```python
from build123d import *

# Parameters (mm, degrees)
ESBO_O1_W                = 50
ESBO_O1_H                = 62
RESSALTO_EXTRUS_O2_DEPTH = 6
ESBO_O3_W                = 10
ESBO_O3_H                = 6
CORTE_EXTRUS_O1_DEPTH    = 6
ESBO_O4_W                = 10
ESBO_O4_H                = 6
CORTE_EXTRUS_O2_DEPTH    = 6
ESBO_O5_W                = 6
ESBO_O5_H                = 10
CORTE_EXTRUS_O3_DEPTH    = 6


with BuildPart() as part:
    # Esboço1 → Ressalto-extrusão2 (new body)
    with BuildSketch(Plane(origin=(0, 0, 0), x_dir=(1, 0, 0), z_dir=(0, 1, 0))):
        Rectangle(ESBO_O1_W, ESBO_O1_H)
    extrude(amount=RESSALTO_EXTRUS_O2_DEPTH)

    # Esboço3 → Corte-extrusão1 (cut)
    with BuildSketch(Plane.XY.offset(31)):
        with Locations((0, 3)):
            Rectangle(ESBO_O3_W, ESBO_O3_H)
    extrude(amount=-CORTE_EXTRUS_O1_DEPTH, mode=Mode.SUBTRACT)

    # Esboço4 → Corte-extrusão2 (cut)
    with BuildSketch(Plane(origin=(0, 0, -31), x_dir=(-1, 0, 0), z_dir=(0, 0, -1))):
        with Locations((0, 3)):
            Rectangle(ESBO_O4_W, ESBO_O4_H)
    extrude(amount=-CORTE_EXTRUS_O2_DEPTH, mode=Mode.SUBTRACT)

    # Esboço5 → Corte-extrusão3 (cut)
    with BuildSketch(Plane(origin=(0, 6, 0), x_dir=(1, 0, 0), z_dir=(0, 1, 0))):
        Rectangle(ESBO_O5_W, ESBO_O5_H)
    extrude(amount=-CORTE_EXTRUS_O3_DEPTH, mode=Mode.SUBTRACT)


solid = part.part
```
Model file for the job. Use its own axes, mm. A direction names the side the tool comes from. Give positions to 0.01 mm unless a question says otherwise; leave off trailing zeros. Write each loop counter-clockwise with the first axis right and the second up, starting at its lowest first coordinate (ties: lowest second). Pieces come first, ordered by that corner, then holes. Notation, with made-up numbers: (56.25, 7.5) -> (96.25, 7.5) arc R8 ccw to (96.25, 15.5) -> close; hole circle Ø5 at (-19.75, -13.75). An arc over 180 degrees is marked (long way). Use CSV: the item, a comma, the result in double quotes. Start each with the question number.
1) Pin check, flat tips, straight feed: P1, Ø3, axis at x = -2.5, y = 4.5, coming from the -Z side; P2, Ø1.8, axis at x = 0.5, y = 2.5, coming from the +Z side. Stop position of each tip, or through.
2) Tool access for faces 1 (the flat face through (5, 3, -28)), 2 (the flat face through (0, 3, -5)), 3 (the flat face through (5, 3, 28)): list every direction of +Z, -Z, +X, -X, +Y, -Y with a clear straight run to the whole face (end or side of a thin tool).
3) Cut at A-A on z = -4. List the corners of the cut face in (x, y).
4) Cut at C-C on z = 26. List the corners of the cut face in (x, y).
5) Cut at B-B on y = 2.1. List the corners of the cut face in (x, z).
6) Two-plate mould, pull along X, no slides. Class faces 4 (the flat face through (-25, 3, 0)), 5 (the flat face through (-15, 3, 31)), 6 (the flat face through (0, 3, 25)): released by +X, released by -X, zero draft, split by the parting line, or undercut.
7) Drill centre lines: L1, parallel to Z at x = 1, y = 1.1; L2, parallel to X at y = 2, z = 3.5; L3, parallel to Z at x = -3.5, y = 5.75. Where is each one in solid material? Low to high.
Final values:
1,P1,"stops at z = -25"
1,P2,"stops at z = 25"
2,face 1,"-Z, +Y, -Y"
2,face 2,"+Y, -Y"
2,face 3,"+Z, +Y, -Y"
3,outline,"(-25, 0) -> (-3, 0) -> (-3, 6) -> (-25, 6) -> close; (3, 0) -> (25, 0) -> (25, 6) -> (3, 6) -> close"
4,outline,"(-25, 0) -> (-5, 0) -> (-5, 6) -> (-25, 6) -> close; (5, 0) -> (25, 0) -> (25, 6) -> (5, 6) -> close"
5,outline,"(-25, -31) -> (-5, -31) -> (-5, -25) -> (5, -25) -> (5, -31) -> (25, -31) -> (25, 31) -> (5, 31) -> (5, 25) -> (-5, 25) -> (-5, 31) -> (-25, 31) -> close; hole (-3, -5) -> (3, -5) -> (3, 5) -> (-3, 5) -> close"
6,face 4,"released by -X"
6,face 5,"zero draft"
6,face 6,"undercut"
7,L1,"z = -25 to -5, 5 to 25"
7,L2,"x = -25 to -3, 3 to 25"
7,L3,"z = -25 to 25"
